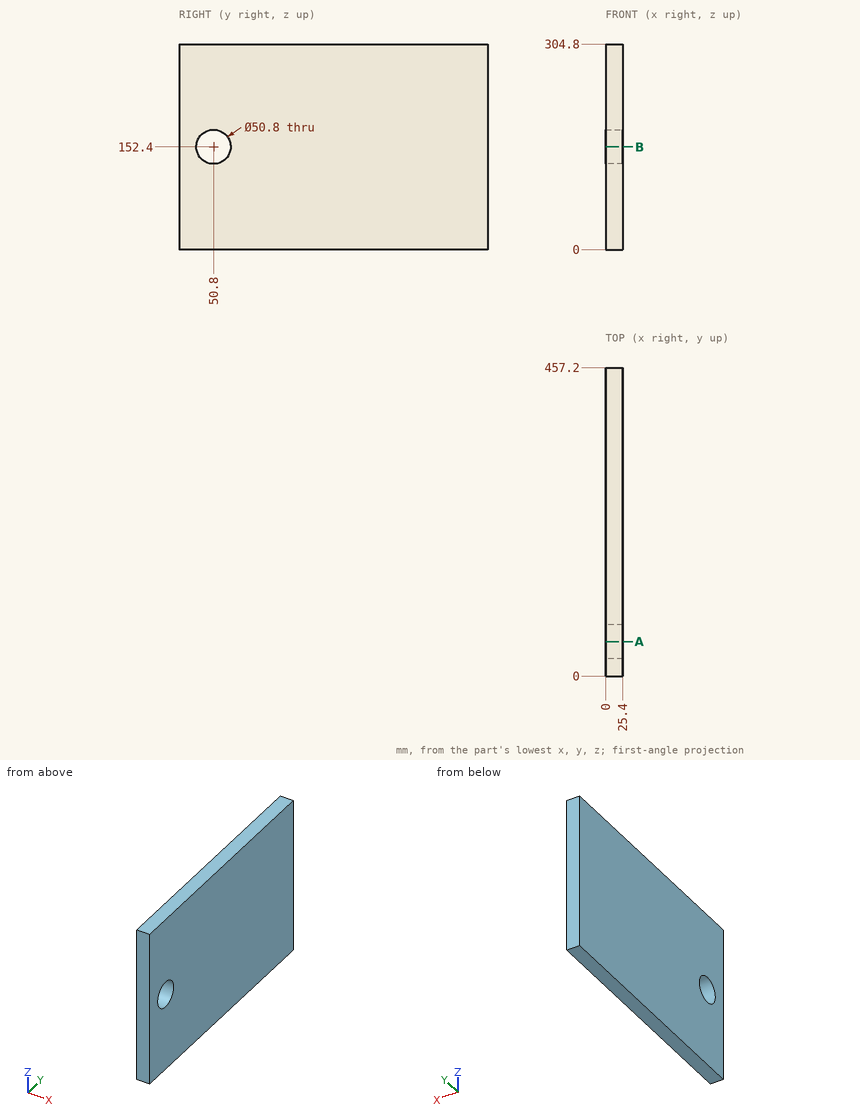
For this review, use the dimensioned drawing (mm, ordinates from the lowest corner) and the shaded views. Give positions to 0.01 mm unless a question says otherwise; leave off trailing zeros. Loops run counter-clockwise (first coordinate to the right, second up) from the corner with the lowest first, then second, coordinate; pieces in that order, holes last.
Item 1: Take a section at A-A, the plane y = 50.8. State the section outline as (x, z) points.
Item 2: For line 1 along Y through (x, z) = (8.5, 152.4); line 2 along Z through (x, y) = (23.75, 30.5); line 3 along Z through (x, y) = (16, 34), list the stretches that pass through material, from the lowest coordinate up.
Item 3: Insertion check: pin 1 (6 mm diameter, centred on x = 21.5, y = 59.5, fed in from -Z). The pin has a flat end and moves straight along its axis. Give the tip position at first contact, or say it passes through.
Item 4: Take a section at B-B, the plane z = 152.4. State the section outline as (x, y) points, and give its area (3 significant figures).
Calculated:
1. outline: (0, 0) - (25.4, 0) - (25.4, 127) - (0, 127) - close; (0, 177.8) - (25.4, 177.8) - (25.4, 304.8) - (0, 304.8) - close
2. line 1: y = 0 to 25.4, 76.2 to 457.2
2. line 2: z = 0 to 137.13, 167.67 to 304.8
2. line 3: z = 0 to 133.35, 171.45 to 304.8
3. pin 1: stops at z = 0
4. outline: (0, 0) - (25.4, 0) - (25.4, 25.4) - (0, 25.4) - close; (0, 76.2) - (25.4, 76.2) - (25.4, 457.2) - (0, 457.2) - close
4. area: 10,300 mm2
